Here's how the part is built. I have some questions about the finished solid (model axes, mm). Face numbers are marked on the shaded views. A direction names the side the tool comes from. Coordinates: 2 decimals unless noted, no trailing zeros. Write each loop counter-clockwise with the first axis right and the second up, starting at its lowest first coordinate (ties: lowest second). Pieces come first, ordered by that corner, then holes. Notation, with made-up numbers: M 19.25,13 L 76.25,13 A20 cw 76.25,23 Z; hole C 4.25,-11.5 d5. An arc over 180 degrees is marked long. Use one line per item in the form item = value. Start each with the question number.
1. I want a section at B-B, the plane z = -22.75. List the corners of the cut face in (x, y) for me.
2. Please list where these lines run through material, in increasing order: line 1 along Y through (x, z) = (-50, -1.4); line 2 along X through (y, z) = (105.5, -24.5); line 3 along Z through (x, y) = (-104, 28). Write a range as [from, to].
3. I want a section at C-C, the plane y = 130. List the corners of the cut face in (x, z) for me.
4. I'm going to push flat-ended pins straight in: pin 1 Ø5 at (x, y) = (-97.5, 106.5) entering from -Z; pin 2 Ø1.5 at (x, y) = (-123.5, 105.5) entering from -Z. Where does each tip first touch, or does it pass through?
5. I want a section at D-D, the plane x = -110. List the corners of the cut face in (y, z) for me.
6. Thinking about a two-plate mould opening in X: for the marked faces 3, 4 and 5, which applies, released by +X, released by -X, zero draft, split by the parting line, or undercut?
7. I want a section at A-A, the plane z = -12.5. Count the separate pieces of the cut face and the enclosed holes in it, plus the area to 3 significant figures.
8. On a 3-axis mill with a long thin cutter (end or side, diameter ignored), from which of +Z, -Z, +X, -X, +Y, -Y can I reach the whole of each face in a straight line? I mean the marked faces 1 and 2. Say none if no direction works.
Autodesk Inventor part; units mm, degrees
ref_plane "YZ Plane" through (0, 0, 0) normal (1, 0, 0) x (0, 1, 0)
ref_plane "XZ Plane" through (0, 0, 0) normal (0, 1, 0) x (-1, 0, 0)
ref_plane "XY Plane" through (0, 0, 0) normal (0, 0, 1) x (1, 0, 0)
sketch "Sketch1" plane through (0, 0, 0) normal (0, 1, 0) x (-1, 0, 0)
  line L0 (0, 0) -> (125, 0)
  line L1 (0, 0) -> (125, 0) construction
  line L2 (125, 0) -> (125, -25)
  line L3 (125, -25) -> (122, -25)
  line L4 (122, -25) -> (122, -3)
  line L5 (122, -3) -> (3, -3)
  line L6 (3, -3) -> (3, -26)
  line L7 (3, -26) -> (0, -26)
  line L8 (0, -26) -> (0, 0)
  dimension "d0" = 125
  dimension "d2" = 25
  dimension "d3" = 90
  dimension "d4" = 90
  dimension "d5" = 3
  dimension "d6" = 22
  dimension "d7" = 119
  dimension "d8" = 90
  dimension "d9" = 23
  dimension "d10" = 90
  dimension "d11" = 3
  dimension "d12" = 90
extrude "Extrusion1" add sketch "Sketch1" along normal blind 150
sketch "Sketch2" plane through (-125, 0, 0) normal (0, 0, 1) x (1, 0, 0)
  circle A0 centre (15, 105) radius 4.25
  circle A1 centre (75, 105) radius 4.25
  circle A2 centre (15, 45) radius 4.25
  circle A3 centre (75, 45) radius 4.25
  line L0 (125, 0) -> (125, 150)
  line L1 (125, 0) -> (0, 0)
  circle A4 centre (45, 75) radius 25
  dimension "d15" = 8.5
  dimension "d16" = 8.5
  dimension "d17" = 8.5
  dimension "d18" = 8.5
  dimension "d19" = 60
  dimension "d20" = 60
  dimension "d21" = 60
  dimension "d22" = 60
  dimension "d23" = 60
  dimension "d24" = 60
  dimension "d25" = 50
  dimension "d26" = 45
  dimension "d27" = 50
  dimension "d28" = 80
  dimension "d29" = 75
extrude "Extrusion2" cut sketch "Sketch2" against normal blind 10
sketch "Sketch3" plane through (-125, 0, -25) normal (-1, 0, 0) x (0, 0, 1)
  circle A0 centre (12.5, 15) radius 2.75
  circle A1 centre (12.5, 135) radius 2.75
  line L0 (25, 0) -> (0, 0)
  line L1 (0, 150) -> (25, 150)
  line L2 (0, 0) -> (0, 150)
  line L3 (25, 0) -> (25, 150)
  circle A2 centre (12.5, 75) radius 2.75
  dimension "d32" = 5.5
  dimension "d33" = 5.5
  dimension "d34" = 15
  dimension "d35" = 15
  dimension "d36" = 12.5
  dimension "d37" = 12.5
  dimension "d38" = 5.5
  dimension "d39" = 12.5
  dimension "d40" = 75
extrude "Extrusion3" cut sketch "Sketch3" against normal blind 154.4625 contours A0 | A1 | A2
sketch "Sketch5" plane through (-125, 0, 0) normal (0, 0, 1) x (1, 0, 0)
  circle A0 centre (20, 130) radius 2.75
  circle A1 centre (105, 130) radius 2.75
  circle A2 centre (105, 20) radius 2.75
  circle A3 centre (20, 20) radius 2.75
  line L0 (0, 0) -> (0, 150)
  line L1 (0, 150) -> (125, 150)
  line L2 (125, 0) -> (125, 150)
  line L3 (125, 0) -> (0, 0)
  dimension "d45" = 5.5
  dimension "d46" = 5.5
  dimension "d47" = 5.5
  dimension "d48" = 5.5
  dimension "d49" = 20
  dimension "d50" = 20
  dimension "d51" = 20
  dimension "d52" = 20
  dimension "d53" = 20
  dimension "d54" = 20
  dimension "d55" = 20
  dimension "d56" = 20
extrude "Extrusion5" cut sketch "Sketch5" against normal through all contours A0 | A1 | A2 | A3
equation "\"d50\" = d49"
equation "\"d51\" = d49"
equation "\"d52\" = d49"
equation "\"d53\" = d49"
equation "\"d54\" = d49"
equation "\"d55\" = d49"
equation "\"d56\" = d49"
properties part number "Pneumatic Connector" material "Aluminum 6061"
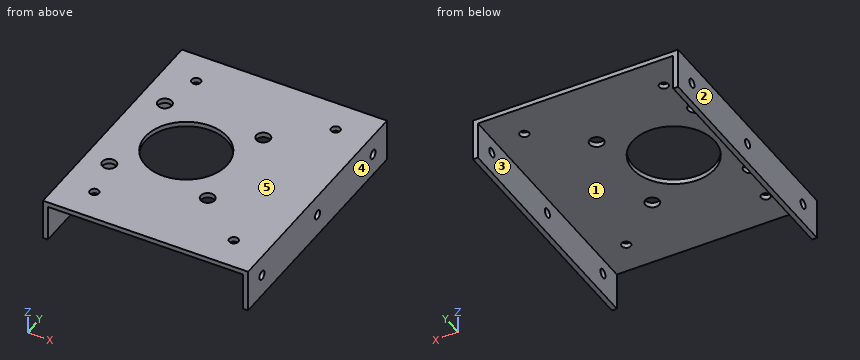
Answer list:
q1.outline = M -125,0 L -122,0 L -122,150 L -125,150 Z; M -3,0 L 0,0 L 0,150 L -3,150 Z
q2.line_1 = [0, 40.75], [49.25, 100.75], [109.25, 150]
q2.line_2 = [-125, -122], [-3, 0]
q2.line_3 = [-3, 0]
q3.outline = M -125,-25 L -122,-25 L -122,-3 L -107.75,-3 L -107.75,0 L -125,0 Z; M -102.25,-3 L -22.75,-3 L -22.75,0 L -102.25,0 Z; M -17.25,-3 L -3,-3 L -3,-26 L 0,-26 L 0,0 L -17.25,0 Z
q4.pin_1 = -3
q4.pin_2 = -25
q5.outline = M 0,-3 L 40.75,-3 L 40.75,0 L 0,0 Z; M 49.25,-3 L 100.75,-3 L 100.75,0 L 49.25,0 Z; M 109.25,-3 L 150,-3 L 150,0 L 109.25,0 Z
q6.face_3 = undercut
q6.face_4 = released by +X
q6.face_5 = zero draft
q7.separate_pieces = 8
q7.enclosed_holes = 0
q7.area = 801 mm²
q8.face_1 = -Z, +Y, -Y
q8.face_2 = +Z, -Z, -X, +Y, -Y
